```python
from build123d import *

# Parameters (mm, degrees)
SKETCH_1_W          = 32
SKETCH_1_H          = 45
EXTRUDE_1_DEPTH     = 16
CUT_EXTRUDE_1_REACH = 33.91
SKETCH_2_R          = 2.25
SKETCH_3_R          = 7.5
EXTRUDE_2_DEPTH     = 30
SKETCH_4_W          = 23
SKETCH_4_H          = 44
EXTRUDE_3_DEPTH     = 14
EXTRUDE_4_DEPTH     = 10
SKETCH_6_R          = 4.527091975
CUT_EXTRUDE_2_DEPTH = 10
SKETCH_7_R          = 4
CUT_EXTRUDE_3_DEPTH = 10


with BuildPart() as part:
    # 草图1 → 凸台-拉伸1 (new body)
    with BuildSketch(Plane.XY):
        Rectangle(SKETCH_1_W, SKETCH_1_H)
    extrude(amount=EXTRUDE_1_DEPTH)

    # 草图2 → 切除-拉伸1 (cut, up to next)
    with BuildSketch(Plane(origin=(0, 0, 0), x_dir=(-1, 0, 0), z_dir=(0, 0, -1)), mode=Mode.PRIVATE) as cut_extrude_1_sk1:
        with Locations((-11, 11.5)):
            Circle(SKETCH_2_R)
    cut_extrude_1_tool1 = extrude(cut_extrude_1_sk1.sketch, amount=-CUT_EXTRUDE_1_REACH, mode=Mode.PRIVATE) & part.part
    # 草图2 → 切除-拉伸1 (cut, up to next)
    with BuildSketch(Plane(origin=(0, 0, 0), x_dir=(-1, 0, 0), z_dir=(0, 0, -1)), mode=Mode.PRIVATE) as cut_extrude_1_sk2:
        with Locations((-11, -8.5)):
            Circle(SKETCH_2_R)
    cut_extrude_1_tool2 = extrude(cut_extrude_1_sk2.sketch, amount=-CUT_EXTRUDE_1_REACH, mode=Mode.PRIVATE) & part.part
    add(cut_extrude_1_tool1.solids().sort_by_distance((11, 11.5, 0))[0], mode=Mode.SUBTRACT)
    add(cut_extrude_1_tool2.solids().sort_by_distance((11, -8.5, 0))[0], mode=Mode.SUBTRACT)

    # 草图3 → 凸台-拉伸2 (add)
    with BuildSketch(Plane(origin=(0, 22.5, 0), x_dir=(1, 0, 0), z_dir=(0, 1, 0))):
        with Locations(Location((6, -8, 0), (0, 0, 90))):
            Circle(SKETCH_3_R)
    extrude(amount=EXTRUDE_2_DEPTH)

    # 草图4 → 凸台-拉伸3 (add)
    with BuildSketch(Plane.XY.offset(16)):
        with Locations((-4.5, 0.5)):
            Rectangle(SKETCH_4_W, SKETCH_4_H)
    extrude(amount=EXTRUDE_3_DEPTH)

    # 草图5 → 凸台-拉伸4 (add)
    with BuildSketch(Plane.XZ.offset(22.5)):
        Polygon((10.501026547, 1.286275746), (14.064769031, 8.541141206), (9.563742484, 15.25486546), (1.498973453, 14.713724254), (-2.064769031, 7.458858794), (2.436257516, 0.74513454), align=None)
    extrude(amount=EXTRUDE_4_DEPTH)

    # 草图6 → 切除-拉伸2 (cut)
    with BuildSketch(Plane.XZ.offset(32.5)):
        with Locations(Location((5.995920122, 7.997264761, 0), (0, 0, 270))):
            Circle(SKETCH_6_R)
    extrude(amount=-CUT_EXTRUDE_2_DEPTH, mode=Mode.SUBTRACT)

    # 草图7 → 切除-拉伸3 (cut)
    with BuildSketch(Plane.ZY.offset(16)):
        with Locations(Location((8, -10.5, 0), (0, 0, 270))):
            Circle(SKETCH_7_R)
    extrude(amount=-CUT_EXTRUDE_3_DEPTH, mode=Mode.SUBTRACT)


solid = part.part
```
Source: CAD feature listing. Evaluate the final solid. Frame: model axes, mm. A direction names the side the tool comes from. Round coordinates to 2 decimals unless told otherwise and drop trailing zeros. Loops run counter-clockwise (first coordinate to the right, second up) from the corner with the lowest first, then second, coordinate; pieces in that order, holes last.
(1) Pull-direction query (X, two-part tool) for faces 1 (the cylindrical face through (12.66, -6.98, 7.89)), 2 (the flat face through (11.846, -27.43, 11.851)), 3 (the flat face through (-5, -21.5, 23)); classes: +X half, -X half, draft (parallel to the pull), parting line (faces both ways), or undercut.
From the geometry:
face 1: undercut
face 2: +X half
face 3: draft
(2) Contact query for flat-ended pins moving along their axis: pin 1 Ø3.5 at (x, y) = (11, 11.5) entering from +Z; pin 2 Ø4.5 at (x, z) = (5.5, 10) entering from -Y; pin 3 Ø7 at (x, y) = (11, -8.5) entering from +Z; pin 4 Ø4 at (x, z) = (-7, 20.5) entering from -Y. Output: stop coordinate, or through.
From the geometry:
pin 1: passes through
pin 2: stops at y = -22.5
pin 3: stops at z = 16
pin 4: stops at y = -21.5
(3) Section query D-D (x = 4.5). Output: boundary loops of the cut face in (y, z), and give its area (3 significant figures).
From the geometry:
outline: (-32.5, 0.88) - (-22.5, 0.88) - (-22.5, 0) - (22.5, 0) - (22.5, 0.65) - (52.5, 0.65) - (52.5, 15.35) - (22.5, 15.35) - (22.5, 30) - (-21.5, 30) - (-21.5, 16) - (-22.5, 16) - (-22.5, 14.92) - (-32.5, 14.92) - (-32.5, 12.27) - (-22.5, 12.27) - (-22.5, 3.72) - (-32.5, 3.72) - close
area: 1,830 mm2
(4) Section query C-C (z = 10). Output: boundary loops of the cut face in (x, y), and give its area (3 significant figures).
From the geometry:
outline: (-16, -22.5) - (-0.82, -22.5) - (-0.82, -32.5) - (1.94, -32.5) - (1.94, -22.5) - (10.06, -22.5) - (10.06, -32.5) - (13.09, -32.5) - (13.09, -22.5) - (16, -22.5) - (16, 22.5) - (13.23, 22.5) - (13.23, 52.5) - (-1.23, 52.5) - (-1.23, 22.5) - (-16, 22.5) - (-16, -7.04) - (-6, -7.04) - (-6, -13.96) - (-16, -13.96) - close; hole circle Ø4.5 at (11, -8.5); hole circle Ø4.5 at (11, 11.5)
area: 1,830 mm2
(5) Section query B-B (x = -14). Output: boundary loops of the cut face in (y, z), and give its area (3 significant figures).
From the geometry:
outline: (-22.5, 0) - (22.5, 0) - (22.5, 30) - (-21.5, 30) - (-21.5, 16) - (-22.5, 16) - close; hole circle Ø8 at (-10.5, 8)
area: 1,290 mm2
(6) Access query for faces 4 (the flat face through (-6, -10, 8)), 5 (the cylindrical face through (-0.324, 37.29, 3.968)), 6 (the flat face through (5.59, -27.43, 14.99)), 7 (the flat face through (6, -22.5, 8)). Directions: +Z, -Z, +X, -X, +Y, -Y. A direction counts if a zero-diameter tool reaches every point of the face in a straight line with its end or side. Return the directions, or none.
From the geometry:
face 4: -X
face 5: +Y
face 6: +Z, -X, -Y
face 7: -Y
(7) Material intervals for probe 1 along Y at (x, z) = (11, 11); probe 2 along Y at (x, z) = (10, 9); probe 3 along Y at (x, z) = (-1, 21.5), sorted ascending.
From the geometry:
probe 1: y = -32.5 to -10.75, -6.25 to 9.25, 13.75 to 52.5
probe 2: y = -22.5 to -10.52, -6.48 to 9.48, 13.52 to 52.5
probe 3: y = -21.5 to 22.5
(8) Section query A-A (y = 11.5). Output: boundary loops of the cut face in (x, z).
From the geometry:
outline: (-16, 0) - (8.75, 0) - (8.75, 16) - (7, 16) - (7, 30) - (-16, 30) - close; (13.25, 0) - (16, 0) - (16, 16) - (13.25, 16) - close
